Geometry check sheet. Reference: drawing and pictorial views, mm from the part's lowest x, y, z. A direction names the side the tool comes from. Round coordinates to 2 decimals unless told otherwise and drop trailing zeros. Loops run counter-clockwise (first coordinate to the right, second up) from the corner with the lowest first, then second, coordinate; pieces in that order, holes last. Notation, with made-up numbers: (69, 55) -> (96, 55) arc R22 ccw to (96, 88) -> close; hole circle Ø6 at (10.25, 72.5). An arc over 180 degrees is marked (long way). Write item = value, one per line.
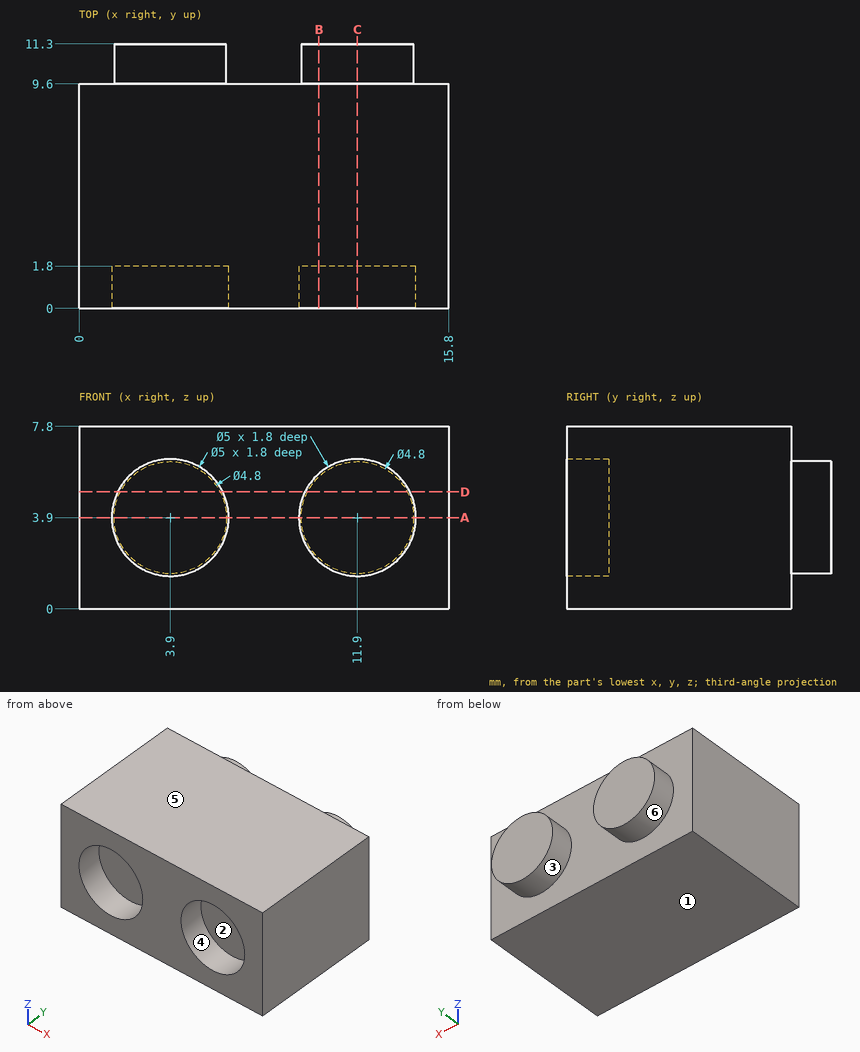
(1) Sectioned sample at D-D, the plane z = 5. Record the cut outline in (x, y) (3 decimals).
Filled sheet:
outline = (0, 0) -> (1.655, 0) -> (1.655, 1.8) -> (6.145, 1.8) -> (6.145, 0) -> (9.655, 0) -> (9.655, 1.8) -> (14.145, 1.8) -> (14.145, 0) -> (15.8, 0) -> (15.8, 9.6) -> (14.033, 9.6) -> (14.033, 11.3) -> (9.767, 11.3) -> (9.767, 9.6) -> (6.033, 9.6) -> (6.033, 11.3) -> (1.767, 11.3) -> (1.767, 9.6) -> (0, 9.6) -> close
(2) Sectioned sample at A-A, the plane z = 3.9. Record the cut outline in (x, y).
Filled sheet:
outline = (0, 0) -> (1.4, 0) -> (1.4, 1.8) -> (6.4, 1.8) -> (6.4, 0) -> (9.4, 0) -> (9.4, 1.8) -> (14.4, 1.8) -> (14.4, 0) -> (15.8, 0) -> (15.8, 9.6) -> (14.3, 9.6) -> (14.3, 11.3) -> (9.5, 11.3) -> (9.5, 9.6) -> (6.3, 9.6) -> (6.3, 11.3) -> (1.5, 11.3) -> (1.5, 9.6) -> (0, 9.6) -> close
(3) Draft check along Z on the marked faces 1, 2 and 3. Enter one of: released by +Z, released by -Z, zero draft, split by the parting line, or undercut.
Filled sheet:
face_1 = released by -Z
face_2 = undercut
face_3 = split by the parting line
(4) Go/stop test with flat-tipped pins: pin 1 Ø2 at (x, z) = (7.5, 3) entering from +Y; pin 2 Ø1.5 at (x, z) = (3.5, 3.5) entering from -Y. Record where each tip stops, or that it passes through.
Filled sheet:
pin_1 = 9.6
pin_2 = 1.8
(5) Material ranges on probe 1 along Z at (x, y) = (3.9, 0.75); probe 2 along Y at (x, z) = (7.25, 3); probe 3 along Y at (x, z) = (11, 3.75), recorded low to high. Write a range as from..to.
Filled sheet:
probe_1 = 0..1.4, 6.4..7.8
probe_2 = 0..9.6
probe_3 = 1.8..11.3
(6) Set-up check for the marked faces 4, 5 and 6: record each of +Z, -Z, +X, -X, +Y, -Y from which the full face is reachable in a straight line by a thin tool's end or side.
Filled sheet:
face_4 = -Y
face_5 = +Z, +X, -X, +Y, -Y
face_6 = +Y
(7) Sectioned sample at B-B, the plane x = 10.25. Record the cut outline in (y, z), and give its area (3 significant figures).
Filled sheet:
outline = (0, 0) -> (9.6, 0) -> (9.6, 2.16) -> (11.3, 2.16) -> (11.3, 5.64) -> (9.6, 5.64) -> (9.6, 7.8) -> (0, 7.8) -> (0, 5.78) -> (1.8, 5.78) -> (1.8, 2.02) -> (0, 2.02) -> close
area = 74.0 mm2
(8) Sectioned sample at C-C, the plane x = 11.9. Record the cut outline in (y, z), and give its area (3 significant figures).
Filled sheet:
outline = (0, 0) -> (9.6, 0) -> (9.6, 1.5) -> (11.3, 1.5) -> (11.3, 6.3) -> (9.6, 6.3) -> (9.6, 7.8) -> (0, 7.8) -> (0, 6.4) -> (1.8, 6.4) -> (1.8, 1.4) -> (0, 1.4) -> close
area = 74.0 mm2
